Job drawing, mm, ordinate dimensions from the low corner. One solid piece. Give positions to 0.01 mm unless a question says otherwise; leave off trailing zeros. Loops run counter-clockwise (first coordinate to the right, second up) from the corner with the lowest first, then second, coordinate; pieces in that order, holes last. Notation, with made-up numbers: (84.5, -38.75) -> (112.5, -38.75) arc R24 cw to (112.5, -5.75) -> close; hole circle Ø4 at (4, 77.5). An arc over 180 degrees is marked (long way). Use one line per item in the form item = value.
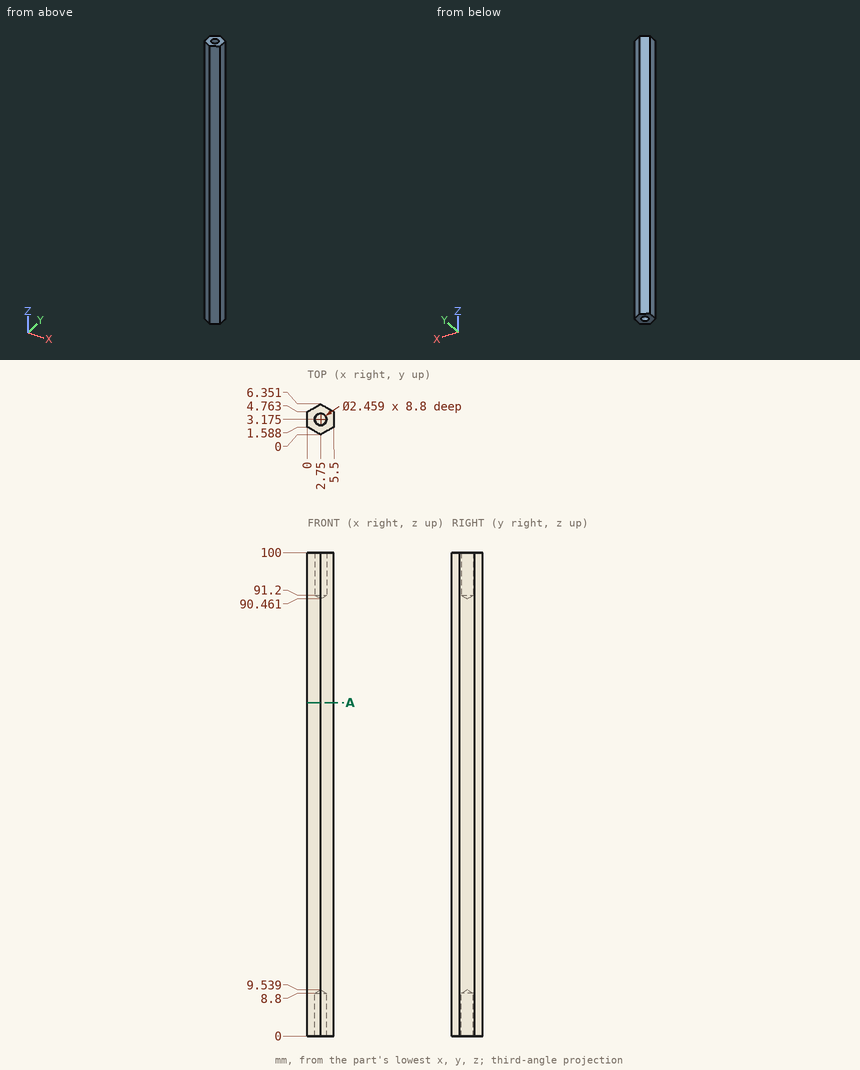
1. Cut at A-A, the plane z = 69. Write the cut outline in (x, y).
Result sheet:
outline = (0, 1.59) -> (2.75, 0) -> (5.5, 1.59) -> (5.5, 4.76) -> (2.75, 6.35) -> (0, 4.76) -> close
2. Drop flat-ended pins along their axis: P1, Ø2, axis at x = 2.75, y = 3.18, coming from the -Z side (1 decimal); P2, Ø1.5, axis at x = 4, z = 70, coming from the -Y side. Give the stop position or say it passes through.
Result sheet:
P1 = 8.9
P2 = 0.29
3. Drill centre lines: line 1 (Y direction, x = 1.75, z = 8.5) (1 decimal); line 2 (X direction, y = 5.25, z = 66) (1 decimal); line 3 (X direction, y = 0.5, z = 89) (1 decimal). Where is each one in solid material? Low to high.
Result sheet:
line_1 = 0.6 to 2.5, 3.9 to 5.8
line_2 = 0.8 to 4.7
line_3 = 1.9 to 3.6
